Autodesk Inventor part; units mm, degrees
ref_plane "Work Plane1" through (0, 0, 2) normal (0, 0, 1) x (1, 0, 0)
ref_plane "YZ Plane" through (0, 0, 0) normal (1, 0, 0) x (0, 1, 0)
ref_plane "XZ Plane" through (0, 0, 0) normal (0, 1, 0) x (-1, 0, 0)
sketch "Sketch1" plane through (0, 0, 0) normal (0, 1, 0) x (-1, 0, 0)
  circle A0 centre (0, 0) radius 1.5
  circle A1 centre (0, -51) radius 1.5
  circle A2 centre (30, -1) radius 1.5
  circle A3 centre (30, -50) radius 1.5
  dimension "d0" = 3
  dimension "d1" = 3
  dimension "d2" = 3
  dimension "d3" = 3
  dimension "d5" = 49
  dimension "d6" = 1
  dimension "d7" = 30
  dimension "d8" = 51
extrude "Extrusion1" add sketch "Sketch1" along normal blind 2.5
sketch "Sketch2" plane through (-30, 2.5, -1) normal (0, 1, 0) x (1, 0, 0)
  circle A0 centre (0, 0) radius 1.5
  line L0 (0, -1.5) -> (30, -2.5)
  circle A1 centre (30, -1) radius 1.5
  line L1 (30, 0.5) -> (0, 1.5)
  circle A2 centre (0, 49) radius 1.5
  circle A3 centre (30, 50) radius 1.5
  line L2 (0, 50.5) -> (29.95, 51.4992)
  line L3 (30, 48.5) -> (0.05, 47.5008)
extrude "Extrusion2" add sketch "Sketch2" along normal blind 45
ref_plane "Work Plane1" through (0, 0, 2) normal (0, 0, 1) x (1, 0, 0)
sketch "Sketch3" plane through (0, 0, 2) normal (0, 0, 1) x (1, 0, 0)
  line L0 (1.5, 0) -> (1.5, 47.5)
  line L1 (1.5, 10) -> (-31.5, 43)
  line L2 (-31.5, 0) -> (-31.5, 47.5)
  line L3 (1.5, 0) -> (-1.5, 0)
  line L4 (-31.5, 43) -> (-31.5, 47.5)
  line L5 (-31.5, 0) -> (-31.5, 47.5)
  line L6 (1.5, 47.5) -> (1.5, 10)
  line L7 (1.5, 47.5) -> (-31.5, 47.5)
  line L8 (0, 2.5) -> (-29.9001, 2.5)
  line L9 (-1.5, 2.5) -> (-28, 2.5)
  line L10 (-28, 2.5) -> (-11.9749, 18.5251)
  line L11 (-11.9749, 18.5251) -> (-1.5, 2.5)
  line L12 (-28.5, 6.9497) -> (-14.4497, 21)
  line L13 (-14.4497, 21) -> (-28.5, 35.0503)
  line L14 (-31.5, 0) -> (-31.5, 47.5)
  line L15 (-10.0429, 18.9973) -> (-1.5, 5.5)
  line L16 (-1.5, 5.5) -> (-1.5, 10.1716)
  line L17 (-1.5, 10.1716) -> (-10.0429, 18.9973)
  line L18 (-28.5, 35.0503) -> (-28.5, 6.9497)
  point P0 (0, 0)
  point P1 (-15, 26.5)
  point P2 (-31.5, 38.0503)
  point P3 (-31.5, 3.9497)
  dimension "d14" = 45
  dimension "d15" = 10
  dimension "d18" = 3.5
  dimension "d19" = 3.5
  dimension "d20" = 3.5
  dimension "d21" = 3.5
  dimension "d22" = 45
  dimension "d23" = 3
  dimension "d24" = 1.8
  dimension "d25" = 3
  dimension "d26" = 2
  dimension "d27" = 12.2831
  dimension "d28" = 3
extrude "Extrusion3" cut sketch "Sketch3" against normal through all
sketch "Sketch4" plane through (0, 0, 2) normal (0, 0, 1) x (1, 0, 0)
  line L0 (1.5, 0) -> (-1.5, 0)
  line L1 (-31.5, 0) -> (-31.5, 43)
  line L2 (1.5, 0) -> (-31.5, 0)
  line L3 (-31.5, 0) -> (-31.5, 43)
  line L4 (-31.5, 43) -> (1.5, 43)
  line L5 (1.5, 43) -> (1.5, 0)
  point P0 (0, 0)
  dimension "d29" = 43
extrude "Extrusion4" cut sketch "Sketch4" against normal blind 10
properties part number "ControlPanel_Middle"
Geometry: final body of the model. Coordinates: model frame, mm. A direction names the side the tool comes from. Give positions to 0.01 mm unless a question says otherwise; leave off trailing zeros. Write each loop counter-clockwise with the first axis right and the second up, starting at its lowest first coordinate (ties: lowest second). Pieces come first, ordered by that corner, then holes.
1. Section query D-D, the plane y = 8. Return loops of the section in (x, z).
2. Pin query (flat end, axial travel): P1, Ø2, axis at x = -11.5, z = -50, coming from the +Y side; P2, Ø1.5, axis at x = -16, z = -50.5, coming from the -Y side; P3, Ø1.5, axis at y = 29.5, z = -51.5, coming from the -X side. Return the tip coordinate at first contact, or that it passes through.
3. Section query A-A, the plane y = 12.5. Return loops of the section in (x, z).
4. Section query C-C, the plane y = 22. Return loops of the section in (x, z), then the cut area to 3 significant figures.
5. Draft query along Y for faces 1 (the cylindrical face through (-31.41, 21.2, -49.49)), 2 (the flat face through (-5.83, 12.34, -50.78)), 3 (the flat face through (-28.3, 2.5, -50.1)), 4 (the flat face through (-28.5, 21, -50)). Return one class per face: released by +Y, released by -Y, zero draft, split by the parting line, or undercut.
6. Line query: probe 1 along X at (y, z) = (18, -50); probe 2 along X at (y, z) = (18, -51.2); probe 3 along Y at (x, z) = (-7.5, -51.35). Output: solid intervals per line, ascending.
7. Reachability of faces 5 (the flat face through (-21.57, 13.88, -50.26)), 6 (the flat face through (-6.81, 10.62, -50.75)), 7 (the flat face through (-1.14, 2.5, -49.77)) from +Z, -Z, +X, -X, +Y, -Y: full face, straight path, thin tool, end or side. Return the list, or none.
8. Section query B-B, the plane x = -6.5. Return loops of the section in (y, z), then the cut area to 3 significant figures.
Computed:
1. outline: (-30, -51.5) - (-28.5, -51.55) - (-28.5, -48.55) - (-29.95, -48.5) arc R1.5 ccw (long way) to start; (-27.45, -51.59) - (-22.5, -51.75) - (-22.5, -48.75) - (-27.45, -48.58) - close; (-5.1, -52.33) - (-3.08, -52.4) - (-3.08, -49.4) - (-5.1, -49.33) - close; (-1.5, -52.45) - (-0.05, -52.5) arc R1.5 ccw (long way) to (0, -49.5) - (-1.5, -49.45) - close
2. P1: stops at y = 24
2. P2: stops at y = 13.75
2. P3: stops at x = -31.3
3. outline: (-30, -51.5) - (-28.5, -51.55) - (-28.5, -48.55) - (-29.95, -48.5) arc R1.5 ccw (long way) to start; (-22.95, -51.74) - (-18, -51.9) - (-18, -48.9) - (-22.95, -48.73) - close; (-8.04, -52.23) - (-5.93, -52.3) - (-5.93, -49.3) - (-8.04, -49.23) - close; (-3.75, -52.38) - (-1, -52.47) - (-1, -49.47) - (-3.75, -49.37) - close
4. outline: (-30, -51.5) - (-28.5, -51.55) - (-28.5, -48.55) - (-29.95, -48.5) arc R1.5 ccw (long way) to start; (-15.45, -51.99) - (-10.5, -52.15) - (-10.5, -49.15) - (-15.45, -48.98) - close
4. area: 22.9 mm2
5. face 1: zero draft
5. face 2: undercut
5. face 3: released by -Y
5. face 4: undercut
6. probe 1: x = -31.5 to -28.5, -17.45 to -12.5, -11.63 to -9.41, -9.08 to -6.5
6. probe 2: x = -30.9 to -28.5, -17.45 to -12.5, -11.63 to -9.41, -9.08 to -6.5
6. probe 3: y = 11.68 to 14.98, 16.37 to 19
7. face 5: +Z, -Z
7. face 6: +Z, -Z, -Y
7. face 7: +Z, -Y
8. outline: (10.15, -52.28) - (13.4, -52.28) - (13.4, -49.28) - (10.15, -49.28) - close; (15.34, -52.28) - (18, -52.28) - (18, -49.28) - (15.34, -49.28) - close
8. area: 17.7 mm2
